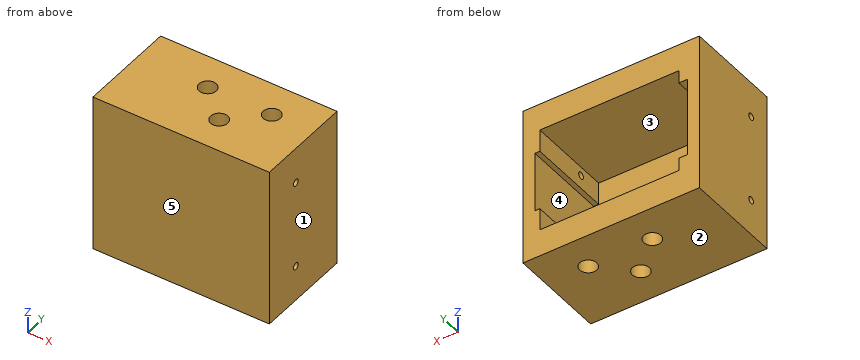
```python
from build123d import *

# Parameters (mm, degrees)
SKETCH1_W           = 41.25
SKETCH1_H           = 37.25
BOSS_EXTRUDE1_DEPTH = 23
CUT_EXTRUDE1_DEPTH  = 20
SKETCH3_R           = 0.8
CUT_EXTRUDE2_DEPTH  = 3.95
SKETCH4_R           = 0.8
CUT_EXTRUDE3_DEPTH  = 4.8
SKETCH5_R           = 2
CUT_EXTRUDE4_DEPTH  = 5.5


with BuildPart() as part:
    # Sketch1 → Boss-Extrude1 (new body)
    with BuildSketch(Plane(origin=(0, 0, 0), x_dir=(1, 0, 0), z_dir=(0, 1, 0))):
        with Locations((20.625, 18.625)):
            Rectangle(SKETCH1_W, SKETCH1_H)
    extrude(amount=BOSS_EXTRUDE1_DEPTH)

    # Sketch2 → Cut-Extrude1 (cut)
    with BuildSketch(Plane(origin=(0, 23, 0), x_dir=(1, 0, 0), z_dir=(0, 1, 0))):
        Polygon((37.3, 30.875), (4.8, 30.875), (4.8, 27.875), (2.8, 27.875), (2.8, 9.375), (4.8, 9.375), (4.8, 6.375), (37.3, 6.375), (37.3, 11.575), (38.45, 11.575), (38.45, 25.675), (37.3, 25.675), align=None)
    extrude(amount=-CUT_EXTRUDE1_DEPTH, mode=Mode.SUBTRACT)

    # Sketch3 → Cut-Extrude2 (cut)
    with BuildSketch(Plane.ZY.offset(-37.3)):
        with Locations((-28.925, 9)):
            Circle(SKETCH3_R)
        with Locations((-8.425, 9)):
            Circle(SKETCH3_R)
    extrude(amount=-CUT_EXTRUDE2_DEPTH, mode=Mode.SUBTRACT)

    # Sketch4 → Cut-Extrude3 (cut)
    with BuildSketch(Plane(origin=(4.8, 0, 0), x_dir=(0, 0, -1), z_dir=(1, 0, 0))):
        with Locations((28.875, 5.4)):
            Circle(SKETCH4_R)
        with Locations((8.375, 5.4)):
            Circle(SKETCH4_R)
    extrude(amount=-CUT_EXTRUDE3_DEPTH, mode=Mode.SUBTRACT)

    # Sketch5 → Cut-Extrude4 (cut)
    with BuildSketch(Plane.XY):
        with Locations((16.5, 15)):
            Circle(SKETCH5_R)
        with Locations((31.5, 15)):
            Circle(SKETCH5_R)
        with Locations((24, 8)):
            Circle(SKETCH5_R)
    cut_extrude4 = extrude(amount=-CUT_EXTRUDE4_DEPTH, mode=Mode.SUBTRACT)

    # Mirror1: Cut-Extrude4 across plane
    add(cut_extrude4.mirror(Plane.XY.offset(-18.625)), mode=Mode.SUBTRACT)


solid = part.part
```
The listing builds one solid part. Answer for the finished solid, in the listing's coordinates (mm). Face numbers are marked on the shaded views. A direction names the side the tool comes from. Give positions to 0.01 mm unless a question says otherwise; leave off trailing zeros. Loops run counter-clockwise (first coordinate to the right, second up) from the corner with the lowest first, then second, coordinate; pieces in that order, holes last. Notation, with made-up numbers: (-40, 41) - (-34, 41) arc R9 cw to (-34, 56) - close; hole circle Ø11 at (27, 53.25). An arc over 180 degrees is marked (long way). Return JSON: item names as keys, results as strings. Group by question number.
1. Find section C-C (y = 5.4). Write down the section's boundary in (x, z) (3 decimals).
2. Find section B-B (z = -8.5). Write down the section's boundary in (x, y).
3. Which of the six approach directions +Z, -Z, +X, -X, +Y, -Y give full straight-line access (tool end or side, diameter ignored) to the marked faces 4 and 5?
4. Find section A-A (y = 18.25). Write down the section's boundary in (x, z) (3 decimals), then the cut area to 3 significant figures.
5. Find section D-D (x = 30.5). Write down the section's boundary in (y, z) (3 decimals).
6. Straight lines are drawn through the part: line 1 (Z direction, x = 28.5, y = 16) (3 decimals); line 2 (X direction, y = 11.25, z = -25); line 3 (X direction, y = 21, z = -28.5). For each, find the intervals that lie inside material, in ascending order. Write a range as [from, to].
7. Determine the mould class of the marked faces 1, 2 and 3 for opening direction X: pulls with the +X half, pulls with the -X half, needs draft (parallel to the pull), parting line crosses it, or undercut.
8. Given pin 1 Ø10 at (x, z) = (16.5, -26.5) entering from +Y; pin 2 Ø19.5 at (x, z) = (27.5, -17.5) entering from +Y; pin 3 Ø1.2 at (x, y) = (17.5, 15.5) entering from -Z, each flat-ended and moving along its own axis, determine where each tip first touches the part or whether it passes through.
Verdict:
{
 "1": {"outline": "(0, -37.25) - (41.25, -37.25) - (41.25, 0) - (0, 0) - (0, -7.575) - (4.8, -7.575) - (4.8, -6.375) - (37.3, -6.375) - (37.3, -11.575) - (38.45, -11.575) - (38.45, -25.675) - (37.3, -25.675) - (37.3, -30.875) - (4.8, -30.875) - (4.8, -29.675) - (0, -29.675) - close; (0, -28.075) - (4.8, -28.075) - (4.8, -27.875) - (2.8, -27.875) - (2.8, -9.375) - (4.8, -9.375) - (4.8, -9.175) - (0, -9.175) - close"},
 "2": {"outline": "(0, 0) - (41.25, 0) - (41.25, 8.2) - (37.3, 8.2) - (37.3, 3) - (4.8, 3) - (4.8, 4.61) - (0, 4.61) - close; (0, 6.19) - (4.8, 6.19) - (4.8, 23) - (0, 23) - close; (37.3, 9.8) - (41.25, 9.8) - (41.25, 23) - (37.3, 23) - close"},
 "3": {"face 4": "+Y", "face 5": "+Z, -Z, +X, -X, -Y"},
 "4": {"outline": "(0, -37.25) - (41.25, -37.25) - (41.25, 0) - (0, 0) - close; hole (2.8, -27.875) - (4.8, -27.875) - (4.8, -30.875) - (37.3, -30.875) - (37.3, -25.675) - (38.45, -25.675) - (38.45, -11.575) - (37.3, -11.575) - (37.3, -6.375) - (4.8, -6.375) - (4.8, -9.375) - (2.8, -9.375) - close", "area": "687 mm^2"},
 "5": {"outline": "(0, -37.25) - (13.268, -37.25) - (13.268, -31.75) - (16.732, -31.75) - (16.732, -37.25) - (23, -37.25) - (23, -30.875) - (3, -30.875) - (3, -6.375) - (23, -6.375) - (23, 0) - (16.732, 0) - (16.732, -5.5) - (13.268, -5.5) - (13.268, 0) - (0, 0) - close"},
 "6": {"line 1": "z = [-37.25, -30.875], [-6.375, 0]", "line 2": "x = [0, 2.8], [38.45, 41.25]", "line 3": "x = [0, 4.8], [37.3, 41.25]"},
 "7": {"face 1": "pulls with the +X half", "face 2": "needs draft", "face 3": "undercut"},
 "8": {"pin 1": "stops at y = 23", "pin 2": "stops at y = 3", "pin 3": "stops at z = -31.75"}
}
